Check sheet for the modelled part. Datum: model origin and axes. Units: mm. Give positions to 0.01 mm unless a question says otherwise; leave off trailing zeros. Order: outer loops, then holes, each group sorted by start corner. A loop starts at its lowest first (then second) coordinate and runs counter-clockwise, first axis right, second up. Notation, with made-up numbers: (83.5, 83.5) - (108.5, 83.5) arc R38 ccw to (108.5, 121.5) - close; hole circle Ø9 at (-31, 77.5). An arc over 180 degrees is marked (long way). Answer in a Markdown table with one row per item.
from build123d import *

# Parameters (mm, degrees)
F0_W     = 725
F0_H     = 12
F1_DEPTH = 528
F2_W     = 6
F2_H     = 6
F3_DEPTH = 725.001
F4_W     = 6
F4_H     = 6
F5_DEPTH = 528.001


with BuildPart() as f1:
    # F0 (on Front) → F1 (new body)
    with BuildSketch(Plane.XZ):
        with Locations((362.5, 6)):
            Rectangle(F0_W, F0_H)
    extrude(amount=F1_DEPTH)

    # F2 (on Right) → F3 (cut, through all)
    with BuildSketch(Plane.YZ):
        with Locations((-525, 3)):
            Rectangle(F2_W, F2_H)
        with Locations((-3, 3)):
            Rectangle(F2_W, F2_H)
    extrude(amount=F3_DEPTH, mode=Mode.SUBTRACT)

    # F4 (on Front) → F5 (cut, through all)
    with BuildSketch(Plane.XZ):
        with Locations((3, 3)):
            Rectangle(F4_W, F4_H)
        with Locations((722, 3)):
            Rectangle(F4_W, F4_H)
    extrude(amount=F5_DEPTH, mode=Mode.SUBTRACT)


solid = f1.part
(1) Thickness scan on L1, parallel to Y at x = 243, z = 2.25; L2, parallel to X at y = -323, z = 1.75. Record the ranges inside material, lowest first.
Geometry says:
| item | result |
|---|---|
| L1 | -522 to -6 |
| L2 | 6 to 719 |
(2) Cross-section at A-A, the plane z = 2. Record the cut outline in (x, y).
Geometry says:
| item | result |
|---|---|
| outline | (6, -522) - (719, -522) - (719, -6) - (6, -6) - close |
(3) Gauge pin test, flat ends, axial feed: P1, Ø5, axis at x = 226.5, z = 3, coming from the +Y side; P2, Ø6.5, axis at x = 498, z = 2, coming from the -Y side; P3, Ø1.8, axis at y = -210.5, z = 3.5, coming from the +X side. Record the tip position at first contact, or that the pin passes through.
Geometry says:
| item | result |
|---|---|
| P1 | y = -6 |
| P2 | y = -522 |
| P3 | x = 719 |
